Autodesk Inventor part; units mm, degrees
ref_plane "YZ Plane" through (0, 0, 0) normal (1, 0, 0) x (0, 1, 0)
ref_plane "XZ Plane" through (0, 0, 0) normal (0, 1, 0) x (-1, 0, 0)
ref_plane "XY Plane" through (0, 0, 0) normal (0, 0, 1) x (1, 0, 0)
sketch "Skizze1" plane through (0, 0, 0) normal (0, 0, 1) x (1, 0, 0)
  line L0 (-18, 43.5) -> (18, 43.5)
  line L1 (25, 36.5) -> (25, -36.5)
  line L2 (18, -43.5) -> (-18, -43.5)
  line L3 (-25, -36.5) -> (-25, 36.5)
  line L4 (-18, 43.5) -> (-18, 36.5)
  line L5 (-18, 36.5) -> (-25, 36.5)
  line L6 (18, 43.5) -> (18, 36.5)
  line L7 (18, 36.5) -> (25, 36.5)
  line L8 (-18, -43.5) -> (-18, -36.5)
  line L9 (-18, -36.5) -> (-25, -36.5)
  line L10 (18, -43.5) -> (18, -36.5)
  line L11 (18, -36.5) -> (25, -36.5)
  line L12 (0, 60.9) -> (0, -60.9)
  line L13 (-35, 0) -> (35, 0)
  point P0 (0, 0)
  dimension "d6" = 87
  dimension "d7" = 50
  dimension "d8" = 7
  dimension "d9" = 7
extrude "Extrusion1" add sketch "Skizze1" along normal blind 10
sketch "Skizze2" plane through (0, 0, 10) normal (0, 0, 1) x (1, 0, 0)
  line L0 (-18, -43.5) -> (18, -43.5)
  line L1 (18, -43.5) -> (18, -36.5)
  line L2 (18, -36.5) -> (25, -36.5)
  line L3 (25, -36.5) -> (25, 36.5)
  line L4 (25, 36.5) -> (18, 36.5)
  line L5 (18, 36.5) -> (18, 43.5)
  line L6 (18, 43.5) -> (-18, 43.5)
  line L7 (-18, 43.5) -> (-18, 36.5)
  line L8 (-18, 36.5) -> (-25, 36.5)
  line L9 (-25, 36.5) -> (-25, -36.5)
  line L10 (-25, -36.5) -> (-18, -36.5)
  line L11 (-18, -36.5) -> (-18, -43.5)
  line L12 (-23.5, 43.5) -> (-21.5, 43.5)
  line L13 (-21.5, 43.5) -> (-21.5, -43.5)
  line L14 (-21.5, -43.5) -> (-23.5, -43.5)
  line L15 (-23.5, -43.5) -> (-23.5, 43.5)
  line L16 (-18, -43.5) -> (18, -43.5)
  point P0 (0, 0)
  dimension "d12" = 1.5
  dimension "d13" = 2
extrude "Extrusion2" cut sketch "Skizze2" against normal blind 8 contours L13 L14 L15 L10 | L10 L15 L8 L13 | L8 L15 L12 L13
pattern_linear "Rechteckige Anordnung1" count 16 spacing 3 along (1, 0, 0) of "Extrusion2"
properties part number "Jetson Kühlkörper Original" material "Aluminium 6061"
For this review, take the finished solid that the model builds, in its own axes (mm). A direction names the side the tool comes from. Coordinates: 2 decimals unless noted, no trailing zeros. Order: outer loops, then holes, each group sorted by start corner. A loop starts at its lowest first (then second) coordinate and runs counter-clockwise, first axis right, second up. Notation, with made-up numbers: (89, 67) - (145, 67) arc R21 ccw to (145, 82) - close; hole circle Ø3 at (77.5, 35.25). An arc over 180 degrees is marked (long way). Answer as CSV lines item,"result". Start each with the question number.
1) Draft analysis for pull direction X (two halves, no side actions). For faces 1 (the flat face through (-18, 40, 5)), 2 (the flat face through (-21, 36.5, 4)), 3 (the flat face through (-23.5, -1, 6)), state which applies: +X half, -X half, draft (parallel to the pull), parting line (faces both ways), or undercut.
2) To check wall thickness, follow line 1 along Z through (x, y) = (-14, -1). State the ranges of the line that lie inside material, in increasing order. Write a range as [from, to].
3) Add section B-B (z = 8.75). Count the separate pieces of the cut face and the enclosed holes in it, then the cut area to 3 significant figures.
4) Add section A-A (z = 1). State the section outline as (x, y) points.
5) Machinability: for faces 4 (the flat face through (-18, -40, 5)), 5 (the flat face through (25, 1, 5)), 6 (the flat face through (9.5, -1, 6)), which of the approach directions +Z, -Z, +X, -X, +Y, -Y give a long, thin tool a straight path to every point of the face, cutting with its end or side? Answer none if there is none.
6) Add section C-C (x = 7.5). State the section outline as (y, z) points.
7) Insertion check: P1, Ø3.5, axis at y = 40.5, z = 7, coming from the -X side; P2, Ø0.6, axis at x = 22, y = 8.5, coming from the +Z side; P3, Ø5.5, axis at x = -23, z = 6, coming from the +Y side. Each pin has a flat end and moves straight along its axis. Give the tip position at first contact, or say it passes through.
Result:
1,face 1,"-X half"
1,face 2,"draft"
1,face 3,"undercut"
2,line 1,"[0, 2]"
3,separate pieces,"17"
3,enclosed holes,"0"
3,area,"1,480 mm^2"
4,outline,"(-25, -36.5) - (-18, -36.5) - (-18, -43.5) - (18, -43.5) - (18, -36.5) - (25, -36.5) - (25, 36.5) - (18, 36.5) - (18, 43.5) - (-18, 43.5) - (-18, 36.5) - (-25, 36.5) - close"
5,face 4,"+Z, -Z, -X, -Y"
5,face 5,"+Z, -Z, +X, +Y, -Y"
5,face 6,"+Z, +Y, -Y"
6,outline,"(-43.5, 0) - (43.5, 0) - (43.5, 2) - (-43.5, 2) - close"
7,P1,"x = -18"
7,P2,"z = 2"
7,P3,"y = 36.5"
